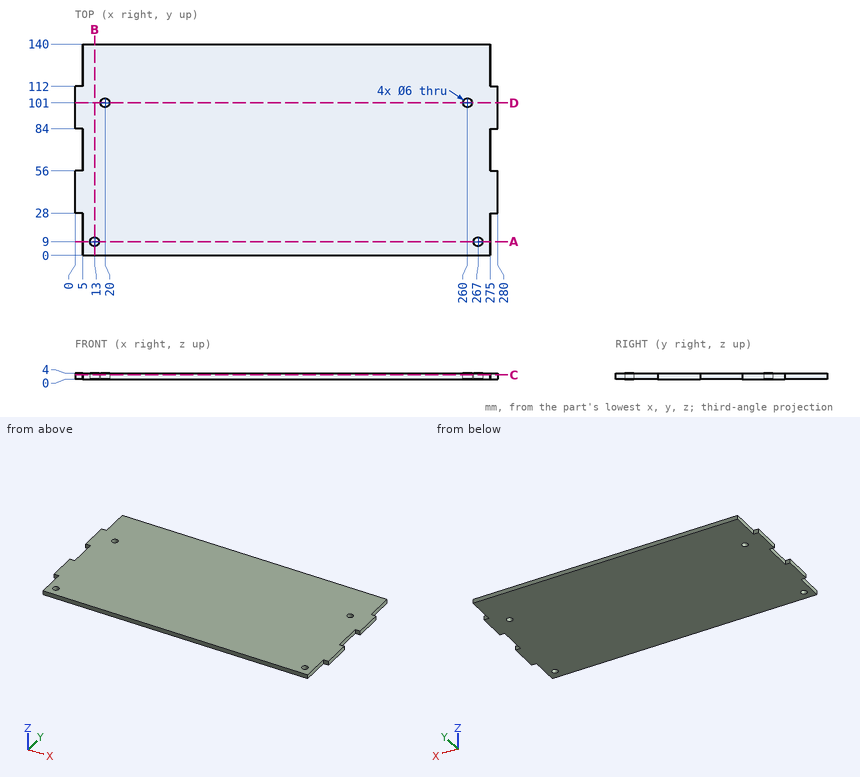
Part print with two shaded views. Sizes in mm from the minimum x, y, z corner. Coordinates: 2 decimals unless noted, no trailing zeros. Write each loop counter-clockwise with the first axis right and the second up, starting at its lowest first coordinate (ties: lowest second). Pieces come first, ordered by that corner, then holes. Notation, with made-up numbers: (-28, 25.5) -> (1, 25.5) arc R15 cw to (1, 30.5) -> close; hole circle Ø2 at (76, -24.5). An arc over 180 degrees is marked (long way). Return JSON: item names as keys, results as strings. Group by question number.
Q1. Drill centre lines: line 1 (Y direction, x = 260, z = 1.45); line 2 (X direction, y = 127.5, z = 1.55); line 3 (Y direction, x = 267, z = 0.9). Where is each one in solid material? Low to high.
Q2. Cut at C-C, the plane z = 2.95. Give the cut face in (x, y).
Q3. Cut at D-D, the plane y = 101. Give the cut face in (x, z), then the cut area to 3 significant figures.
Q4. Cut at B-B, the plane x = 13. Give the cut face in (y, z), then the cut area to 3 significant figures.
Q5. Flat gauge pins, fed straight in: pin 1 (1.2 mm diameter, centred on y = 14, z = 1.5, fed in from +X); pin 2 (2 mm diameter, centred on y = 119.5, z = 1, fed in from -X); pin 3 (2 mm diameter, centred on x = 278, z = 2, fed in from -Y); pin 4 (5 mm diameter, centred on x = 260, y = 101, fed in from +Z). Where does each tip first touch, or does it go through?
Q6. Cut at A-A, the plane y = 9. Give the cut face in (x, z), then the cut area to 3 significant figures.
Returned:
{
 "1": {"line 1": "y = 0 to 98, 104 to 140", "line 2": "x = 5 to 275", "line 3": "y = 0 to 6, 12 to 140"},
 "2": {"outline": "(0, 28) -> (5, 28) -> (5, 0) -> (275, 0) -> (275, 28) -> (280, 28) -> (280, 56) -> (275, 56) -> (275, 84) -> (280, 84) -> (280, 112) -> (275, 112) -> (275, 140) -> (5, 140) -> (5, 112) -> (0, 112) -> (0, 84) -> (5, 84) -> (5, 56) -> (0, 56) -> close; hole circle Ø6 at (13, 9); hole circle Ø6 at (20, 101); hole circle Ø6 at (260, 101); hole circle Ø6 at (267, 9)"},
 "3": {"outline": "(0, 0) -> (17, 0) -> (17, 4) -> (0, 4) -> close; (23, 0) -> (257, 0) -> (257, 4) -> (23, 4) -> close; (263, 0) -> (280, 0) -> (280, 4) -> (263, 4) -> close", "area": "1,070 mm2"},
 "4": {"outline": "(0, 0) -> (6, 0) -> (6, 4) -> (0, 4) -> close; (12, 0) -> (140, 0) -> (140, 4) -> (12, 4) -> close", "area": "536 mm2"},
 "5": {"pin 1": "stops at x = 275", "pin 2": "stops at x = 5", "pin 3": "stops at y = 28", "pin 4": "passes through"},
 "6": {"outline": "(5, 0) -> (10, 0) -> (10, 4) -> (5, 4) -> close; (16, 0) -> (264, 0) -> (264, 4) -> (16, 4) -> close; (270, 0) -> (275, 0) -> (275, 4) -> (270, 4) -> close", "area": "1,030 mm2"}
}
